Verification items for the finished model (mm, model axes). Face numbers are marked on the shaded views. A direction names the side the tool comes from. Coordinates: 2 decimals unless noted, no trailing zeros. Loops run counter-clockwise (first coordinate to the right, second up) from the corner with the lowest first, then second, coordinate; pieces in that order, holes last. Notation, with made-up numbers: M 55,83.5 L 74,83.5 A23 cw 74,92.5 Z; hole C 4.5,1 d5. An arc over 180 degrees is marked long. Write item = value, one per line. Start each with the question number.
```python
from build123d import *

# Parameters (mm, degrees)
SKETCH1_R               = 1.1
BOSS_EXTRUDE1_DEPTH     = 3
FILLET1_R               = 4
CUT_EXTRUDE1_DEPTH      = 10
CUT_EXTRUDE1_DEPTH_BACK = 25.78431964
SKETCH2_W               = 1.2
SKETCH2_H               = 2.5
SKETCH2_W_2             = 3
SKETCH2_H_2             = 1.5
SKETCH2_H_3             = 2
SKETCH3_W               = 26.5
SKETCH3_H               = 5
BOSS_EXTRUDE2_DEPTH     = 3


with BuildPart() as part:
    # Sketch1 → Boss-Extrude1 (new body)
    with BuildSketch(Plane.XY):
        Polygon((-23.05, 8.6), (-23.05, -6.1), (-11.25, -6.1), (-11.25, 6.1), (11.25, 6.1), (11.25, -6.1), (23.05, -6.1), (23.05, 8.6), align=None)
        with Locations((-13.9, 0)):
            Circle(SKETCH1_R, mode=Mode.SUBTRACT)
        with Locations((13.9, 0)):
            Circle(SKETCH1_R, mode=Mode.SUBTRACT)
    extrude(amount=BOSS_EXTRUDE1_DEPTH)

    # Fillet1
    fillet1_edges = [part.edges().sort_by_distance(p)[0] for p in [
        (-23.05, 8.6, 1.5),
        (23.05, 8.6, 1.5),
    ]]
    fillet(fillet1_edges, radius=FILLET1_R)

    # Sketch2 → Cut-Extrude1 (cut, two sides: drawn at the far end of the back side and taken through both)
    with BuildSketch(Plane(origin=(0, 0, 0), x_dir=(-1, 0, 0), z_dir=(0, 0, -1)).offset(-CUT_EXTRUDE1_DEPTH_BACK)):
        with Locations((-20.45, -2.85)):
            Rectangle(SKETCH2_W, SKETCH2_H)
        with Locations((-18.35, -0.85)):
            Rectangle(SKETCH2_W_2, SKETCH2_H_2)
        with Locations((-16.25, -2.85)):
            Rectangle(SKETCH2_W, SKETCH2_H)
        with Locations((-18.35, -2.85)):
            Rectangle(SKETCH2_W_2, SKETCH2_H)
        with Locations((-18.35, -5.1)):
            Rectangle(SKETCH2_W_2, SKETCH2_H_3)
        with Locations((18.35, -0.85)):
            Rectangle(SKETCH2_W_2, SKETCH2_H_2)
        with Locations((16.25, -2.85)):
            Rectangle(SKETCH2_W, SKETCH2_H)
        with Locations((18.35, -2.85)):
            Rectangle(SKETCH2_W_2, SKETCH2_H)
        with Locations((18.35, -5.1)):
            Rectangle(SKETCH2_W_2, SKETCH2_H_3)
        with Locations((20.45, -2.85)):
            Rectangle(SKETCH2_W, SKETCH2_H)
    extrude(amount=CUT_EXTRUDE1_DEPTH + CUT_EXTRUDE1_DEPTH_BACK, mode=Mode.SUBTRACT)

    # Sketch3 → Boss-Extrude2 (add)
    with BuildSketch(Plane(origin=(0, 0, 0), x_dir=(-1, 0, 0), z_dir=(0, 0, -1))):
        with Locations((0, -8.6)):
            Rectangle(SKETCH3_W, SKETCH3_H)
    extrude(amount=-BOSS_EXTRUDE2_DEPTH)


solid = part.part
```
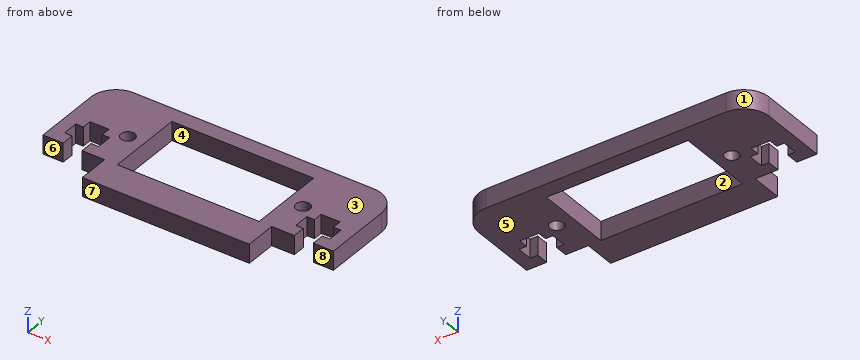
Q1. Scan lines: L1, parallel to X at y = -5, z = 2.85; L2, parallel to X at y = -2.25, z = 0.25; L3, parallel to Y at x = 3, z = 2.1. Record each from-to range of solid material in increasing order. Write a range as [from, to].
Q2. Mould release check, pull along X, two halves, no side actions. Record for the marked faces 1, 2 and 3: +X half, -X half, draft (parallel to the pull), parting line (faces both ways), or undercut.
Q3. Sectioned sample at B-B on y = -5.5. Record the cut outline in (x, z).
Q4. Sectioned sample at A-A on x = 13.9. Record the cut outline in (y, z).
Q5. Gauge pin test, flat ends, axial feed: pin 1 (3 mm diameter, centred on x = -6, y = 6, fed in from +Z); pin 2 (1.3 mm diameter, centred on x = -16.5, z = 2, fed in from -Y); pin 3 (0.9 mm diameter, centred on x = -18.5, z = 1, fed in from -Y). Record the tip position at first contact, or that the pin passes through.
Q6. Set-up check for the marked faces 4, 5, 6, 7 and 8: record each of +Z, -Z, +X, -X, +Y, -Y from which the full face is reachable in a straight line by a thin tool's end or side.
Q7. Sectioned sample at D-D on z = 1.35. Count the separate pieces of the cut face and the enclosed holes in it, plus the area to 3 significant figures.
Q8. Sectioned sample at C-C on x = 5.5. Record the cut outline in (y, z).
Solutions:
q1.L1 = [-23.05, -19.85], [-16.85, -11.25], [11.25, 16.85], [19.85, 23.05]
q1.L2 = [-23.05, -21.05], [-15.65, -11.25], [11.25, 15.65], [21.05, 23.05]
q1.L3 = [-11.1, -6.1], [6.1, 8.6]
q2.face_1 = -X half
q2.face_2 = undercut
q2.face_3 = draft
q3.outline = M -23.05,0 L -19.85,0 L -19.85,3 L -23.05,3 Z; M -16.85,0 L -11.25,0 L -11.25,3 L -16.85,3 Z; M 11.25,0 L 16.85,0 L 16.85,3 L 11.25,3 Z; M 19.85,0 L 23.05,0 L 23.05,3 L 19.85,3 Z
q4.outline = M -6.1,0 L -1.1,0 L -1.1,3 L -6.1,3 Z; M 1.1,0 L 8.6,0 L 8.6,3 L 1.1,3 Z
q5.pin_1 = 3
q5.pin_2 = -6.1
q5.pin_3 = -0.1
q6.face_4 = +Z, -Z
q6.face_5 = -Z, +X, -X, +Y, -Y
q6.face_6 = +Z, -Z, -X, -Y
q6.face_7 = +Z, -Z, +X, -X, -Y
q6.face_8 = +Z, -Z, +X, -Y
q7.separate_pieces = 1
q7.enclosed_holes = 3
q7.area = 473 mm²
q8.outline = M -11.1,0 L -6.1,0 L -6.1,3 L -11.1,3 Z; M 6.1,0 L 8.6,0 L 8.6,3 L 6.1,3 Z
